Work out the finished part from the listing and answer in its coordinate system (mm). A direction names the side the tool comes from. Round coordinates to 2 decimals unless told otherwise and drop trailing zeros. Loops run counter-clockwise (first coordinate to the right, second up) from the corner with the lowest first, then second, coordinate; pieces in that order, holes last. Notation, with made-up numbers: (44, 76) - (93, 76) arc R17 cw to (93, 87) - close; hole circle Ø6 at (1.25, 45.5). An arc over 180 degrees is marked (long way). Return JSON: item names as keys, results as strings.
from build123d import *

# Parameters (mm, degrees)
PAD_DEPTH    = 495
SKETCH001_W  = 18
SKETCH001_H  = 18
POCKET_DEPTH = 138
FILLET_R     = 10


with BuildPart() as part:
    # Sketch → Pad (new body)
    with BuildSketch(Plane.XZ):
        Polygon((138, 0), (0, 0), (0, -20), (-12, -20), (-12, 80), (138, 80), align=None)
    extrude(amount=-PAD_DEPTH)

    # Sketch001 (on Face2 of Pad) → Pocket (cut)
    with BuildSketch(Plane(origin=(138, 0, 0), x_dir=(0, 0, 1), z_dir=(1, 0, 0))):
        with Locations((9, -9)):
            Rectangle(SKETCH001_W, SKETCH001_H)
        with Locations((9, -486)):
            Rectangle(SKETCH001_W, SKETCH001_H)
    extrude(amount=-POCKET_DEPTH, mode=Mode.SUBTRACT)

    # Fillet
    fillet_edges = [part.edges().sort_by_distance(p)[0] for p in [
        (-12, 247.5, 80),
    ]]
    fillet(fillet_edges, radius=FILLET_R)


solid = part.part
1) Section C-C (x = 90.5) is taken. Give the vertices of the cut face in (y, z), and give its area (3 significant figures).
Verdict:
{"outline": "(0, 18) - (18, 18) - (18, 0) - (477, 0) - (477, 18) - (495, 18) - (495, 80) - (0, 80) - close", "area": "39,000 mm2"}
2) Section A-A (z = 6.5) is taken. Give the vertices of the cut face in (x, y).
Verdict:
{"outline": "(-12, 0) - (0, 0) - (0, 18) - (138, 18) - (138, 477) - (0, 477) - (0, 495) - (-12, 495) - close"}
3) Flat-ended cylindrical pins translate along their axes: pin 1 (5 mm diameter, centred on x = 20.5, y = 281.5, fed in from -Z); pin 2 (5.5 mm diameter, centred on x = 90.5, y = 487, fed in from -Z); pin 3 (9 mm diameter, centred on x = 102, z = 6, fed in from +Y). Find the tip coordinate at first contact, or state that the pin passes through.
Verdict:
{"pin 1": "stops at z = 0", "pin 2": "stops at z = 18", "pin 3": "stops at y = 477"}
4) Find the intervals of material crossed by L1, parallel to X at y = 326.5, z = -2; L2, parallel to Z at x = 52.5, y = 207; L3, parallel to Z at x = -3, y = 161.5, in increasing order.
Verdict:
{"L1": "x = -12 to 0", "L2": "z = 0 to 80", "L3": "z = -20 to 79.95"}
5) Section B-B (y = 171.5) is taken. Give the vertices of the cut face in (x, z).
Verdict:
{"outline": "(-12, -20) - (0, -20) - (0, 0) - (138, 0) - (138, 80) - (-2, 80) arc R10 ccw to (-12, 70) - close"}
6) A tool of negligible diameter and unlimited length cuts with its end or side. For faces 1 (the cylindrical face through (-8.99, 250.96, 77.15)), 2 (the flat face through (70, 486, 18)), 3 (the flat face through (70, 244, 0)), 4 (the flat face through (70, 18, 9)), from which of +Z, -Z, +X, -X, +Y, -Y can it reach the whole face along a straight path? Write none if from no direction.
Verdict:
{"face 1": "+Z, -X, +Y, -Y", "face 2": "-Z, +X, +Y", "face 3": "-Z, +X, +Y, -Y", "face 4": "-Z, +X, -Y"}
